Could you check a few things on this model? Use its own coordinates, in mm. A direction names the side the tool comes from. Give positions to 0.01 mm unless a question says otherwise; leave off trailing zeros. Order: outer loops, then holes, each group sorted by start corner. A loop starts at its lowest first (then second) coordinate and runs counter-clockwise, first axis right, second up.
from build123d import *

# Parameters (mm, degrees)
CROQUIS1_R                          = 18.4
SALIENTE_EXTRUIR1_DEPTH             = 90
CROQUIS2_R                          = 3
SALIENTE_EXTRUIR2_DEPTH             = 20
TALADRO_ROSCADO_M3X0_51_D           = 2.5
TALADRO_ROSCADO_M3X0_51_DEPTH       = 8.5
TALADRO_ROSCADO_M3X0_51_CBORE_D     = 3
TALADRO_ROSCADO_M3X0_51_CBORE_DEPTH = 6
TALADRO_ROSCADO_M3X0_51_TIP         = 0.751075774
CROQUIS7_R                          = 6
SALIENTE_EXTRUIR3_DEPTH             = 6.5
CORTAR_EXTRUIR1_DEPTH               = 2
CROQUIS9_W                          = 4.472135954
CROQUIS9_H                          = 10.231682496
CORTAR_EXTRUIR2_DEPTH               = 10


with BuildPart() as part:
    # Croquis1 → Saliente-Extruir1 (new body)
    with BuildSketch(Plane(origin=(0, 0, 0), x_dir=(1, 0, 0), z_dir=(0, 1, 0))):
        with Locations(Location((0, 0, 0), (0, 0, 90))):
            Circle(CROQUIS1_R)
    extrude(amount=SALIENTE_EXTRUIR1_DEPTH)

    # Croquis2 → Saliente-Extruir2 (add)
    with BuildSketch(Plane(origin=(0, 0, 0), x_dir=(-1, 0, 0), z_dir=(0, -1, 0))):
        with Locations(Location((0, 7, 0), (0, 0, 270))):
            Circle(CROQUIS2_R)
    extrude(amount=SALIENTE_EXTRUIR2_DEPTH)

    # Taladro roscado M3x0.51
    with Locations(Plane(origin=(0, 0, 0), x_dir=(-1, 0, 0), z_dir=(0, -1, 0))):
        with Locations((-7.75, -13.423393759), (-15.5, 0), (-7.75, 13.423393759), (7.75, 13.423393759), (15.5, 0), (7.75, -13.423393759)):
            CounterBoreHole(TALADRO_ROSCADO_M3X0_51_D / 2, TALADRO_ROSCADO_M3X0_51_CBORE_D / 2, TALADRO_ROSCADO_M3X0_51_CBORE_DEPTH, depth=TALADRO_ROSCADO_M3X0_51_DEPTH)
            with Locations((0, 0, -(TALADRO_ROSCADO_M3X0_51_DEPTH + TALADRO_ROSCADO_M3X0_51_TIP / 2))):  # 118° drill point
                Cone(0, TALADRO_ROSCADO_M3X0_51_D / 2, TALADRO_ROSCADO_M3X0_51_TIP, mode=Mode.SUBTRACT)

    # Croquis7 → Saliente-Extruir3 (add)
    with BuildSketch(Plane(origin=(0, 0, 0), x_dir=(-1, 0, 0), z_dir=(0, -1, 0))):
        with Locations(Location((0, 7, 0), (0, 0, 270))):
            Circle(CROQUIS7_R)
    extrude(amount=SALIENTE_EXTRUIR3_DEPTH)

    # Croquis8 → Cortar-Extruir1 (cut)
    with BuildSketch(Plane(origin=(0, 0, 0), x_dir=(-1, 0, 0), z_dir=(0, -1, 0))):
        with BuildLine():
            ThreePointArc((-8.481146613, 9.852418593), (0, -13), (8.481146613, 9.852418593))
            ThreePointArc((8.481146613, 9.852418593), (0, -1.947968468), (-8.481146613, 9.852418593))
        make_face()
    extrude(amount=-CORTAR_EXTRUIR1_DEPTH, mode=Mode.SUBTRACT)

    # Croquis9 → Cortar-Extruir2 (cut)
    with BuildSketch(Plane.XZ.offset(20)):
        with Locations((0, 0.115841248)):
            Rectangle(CROQUIS9_W, CROQUIS9_H)
    extrude(amount=-CORTAR_EXTRUIR2_DEPTH, mode=Mode.SUBTRACT)


solid = part.part
Item 1: For faces 4 (the flat face through (0, -20, -8)), 5 (the cylindrical face through (-14, 3, 0)), which set-ups out of +Z, -Z, +X, -X, +Y, -Y let a thin tool reach every point of the face, with its end or its side?
Findings:
face 4: +Z, -Z, +X, -X, -Y
face 5: -Y
Item 2: For pin 1 (5 mm diameter, centred on x = -13, y = 20.5, fed in from +Z); pin 2 (6 mm diameter, centred on x = 12.5, y = 43, fed in from -Z); pin 3 (2.5 mm diameter, centred on x = -8, z = -13, fed in from -Y), each with a flat end and sliding along its axis, tell me the tip position at first contact or that it passes through.
Findings:
pin 1: stops at z = 15.11
pin 2: stops at z = -15.76
pin 3: stops at y = 0
Item 3: Imagine slicing it at B-B on y = 74. List the corners of the cut face in (x, z) for me, then the cut area to 3 significant figures.
Findings:
outline: circle Ø36.8 at (0, 0)
area: 1,060 mm2
Item 4: Imagine slicing it at A-A on x = 0. List the corners of the cut face in (y, z) for me, then the cut area to 3 significant figures.
Findings:
outline: (-20, -10) - (-6.5, -10) - (-6.5, -13) - (0, -13) - (0, -18.4) - (90, -18.4) - (90, 18.4) - (0, 18.4) - (0, 13) - (2, 13) - (2, 1.95) - (0, 1.95) - (0, -1) - (-6.5, -1) - (-6.5, -4) - (-10, -4) - (-10, -5) - (-20, -5) - close
area: 3,440 mm2
Item 5: We'd pull the mould along X, two halves only. Please class faces 1 (the cylindrical face through (8.856, 2.958, 12.41)), 2 (the cylindrical face through (0, -13, -10)), 3 (the flat face through (1, -6.5, -10)): +X half, -X half, draft (parallel to the pull), parting line (faces both ways), or undercut.
Findings:
face 1: undercut
face 2: parting line
face 3: draft
Item 6: Please list where these lines run through material, in increasing order: line 1 along Z through (x, y) = (7, 3); line 2 along Y through (x, z) = (7.5, -6); line 3 along Z through (x, y) = (-15, 3).
Findings:
line 1: z = -17.02 to -14.72, -12.12 to 12.12, 14.72 to 17.02
line 2: y = 0 to 90
line 3: z = -10.66 to -1.41, 1.41 to 10.66
